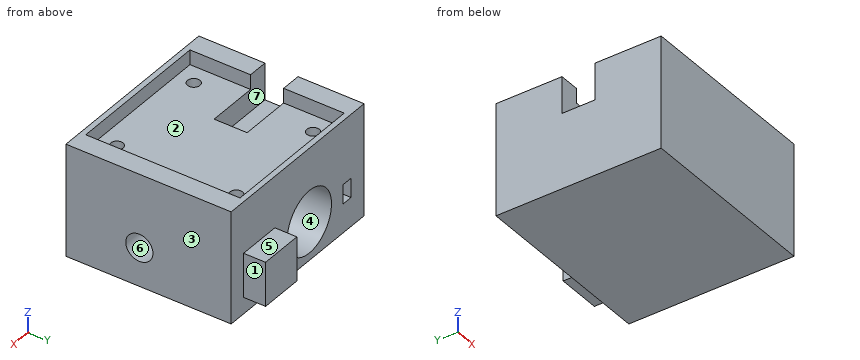
from build123d import *

# Parameters (mm, degrees)
BASE_R                        = 10.5
CUTLURE_TUBE_HOUSING_DEPTH    = 45
SKETCH1_W                     = 51
SKETCH1_H                     = 30.5
DETECTOR_LASER_HOUSING_DEPTH  = 45
CULTURE_SLOT_R                = 8.5
CULTURE_TUBE_SLOT_DEPTH       = 40
LASER_PORT_DEPTH              = 58.662812973
LASER_PORT_DEPTH_BACK         = 16
SKETCH3_R                     = 3.7
CUT_EXTRUDE3_REACH            = 59.663
CUT_EXTRUDE3_END_RADIUS       = 3.7
SKETCH4_W                     = 3
SKETCH4_H                     = 5.25
LED_DISPLAY_SCREW_HOLES_D     = 3.4
LED_DISPLAY_SCREW_HOLES_DEPTH = 20
SKETCH14_W                    = 40
SKETCH14_H                    = 42
CUT_EXTRUDE4_DEPTH            = 4
SKETCH16_W                    = 19.5
SKETCH16_H                    = 9
CUT_EXTRUDE6_DEPTH            = 10
SKETCH17_W                    = 12
SKETCH17_H                    = 12
BOSS_EXTRUDE3_DEPTH           = 6


with BuildPart() as part:
    # Base → Cutlure Tube Housing (new body)
    with BuildSketch(Plane(origin=(0, 0, 0), x_dir=(1, 0, 0), z_dir=(0, 1, 0))):
        with Locations(Location((0, 0, 0), (0, 0, 90))):
            Circle(BASE_R)
    extrude(amount=CUTLURE_TUBE_HOUSING_DEPTH)

    # Sketch1 → Detector+Laser Housing (add)
    with BuildSketch(Plane(origin=(0, 45, 0), x_dir=(1, 0, 0), z_dir=(0, 1, 0))):
        with Locations((4.5, -4.75)):
            Rectangle(SKETCH1_W, SKETCH1_H)
    extrude(amount=-DETECTOR_LASER_HOUSING_DEPTH)

    # Culture Slot → Culture Tube Slot (cut)
    with BuildSketch(Plane(origin=(0, 45, 0), x_dir=(1, 0, 0), z_dir=(0, 1, 0))):
        with Locations(Location((0, 0, 0), (0, 0, 270))):
            Circle(CULTURE_SLOT_R)
    extrude(amount=-CULTURE_TUBE_SLOT_DEPTH, mode=Mode.SUBTRACT)

    # Sketch3 → Laser Port (cut, two sides: drawn at the far end of the back side and taken through both)
    with BuildSketch(Plane(origin=(0, 0, 0), x_dir=(0, 0, -1), z_dir=(1, 0, 0)).offset(-LASER_PORT_DEPTH_BACK)):
        with Locations((0, 20)):
            Circle(SKETCH3_R)
    extrude(amount=LASER_PORT_DEPTH + LASER_PORT_DEPTH_BACK, mode=Mode.SUBTRACT)

    # Cut-Extrude3: up to this cylinder (the profile starts outside it)
    cut_extrude3_end = Plane(origin=(-14.5, 20, 0), z_dir=(1, 0, 0)) * Cylinder(CUT_EXTRUDE3_END_RADIUS, 127.726, mode=Mode.PRIVATE)
    # Sketch4 → Cut-Extrude3 (cut, up to the surface)
    with BuildSketch(Plane(origin=(0, 45, 0), x_dir=(1, 0, 0), z_dir=(0, 1, 0)), mode=Mode.PRIVATE) as cut_extrude3_sk1:
        with Locations((-14.5, 0)):
            Rectangle(SKETCH4_W, SKETCH4_H)
    cut_extrude3_tool1 = extrude(cut_extrude3_sk1.sketch, amount=-CUT_EXTRUDE3_REACH, mode=Mode.PRIVATE) - cut_extrude3_end
    add(cut_extrude3_tool1.solids().sort_by_distance((-14.5, 45, 0))[0], mode=Mode.SUBTRACT)

    # LED display Screw Holes
    with Locations(Plane.XY.offset(20)):
        with Locations((-10.25, 38.75), (-10.25, 6.25), (19.25, 38.75), (19.25, 6.25)):
            Hole(LED_DISPLAY_SCREW_HOLES_D / 2, depth=LED_DISPLAY_SCREW_HOLES_DEPTH)

    # Sketch14 → Cut-Extrude4 (cut)
    with BuildSketch(Plane.XY.offset(20)):
        with Locations((4.5, 22.5)):
            Rectangle(SKETCH14_W, SKETCH14_H)
    extrude(amount=-CUT_EXTRUDE4_DEPTH, mode=Mode.SUBTRACT)

    # Sketch16 → Cut-Extrude6 (cut)
    with BuildSketch(Plane.XY.offset(20)):
        with Locations((-11.25, 22.5)):
            Rectangle(SKETCH16_W, SKETCH16_H)
    extrude(amount=-CUT_EXTRUDE6_DEPTH, mode=Mode.SUBTRACT)

    # Sketch17 → Boss-Extrude3 (add)
    with BuildSketch(Plane(origin=(0, 45, 0), x_dir=(1, 0, 0), z_dir=(0, 1, 0))):
        with Locations((19.25, 0)):
            Rectangle(SKETCH17_W, SKETCH17_H)
    extrude(amount=BOSS_EXTRUDE3_DEPTH)


solid = part.part
Here's how the part is built. I have some questions about the finished solid (model axes, mm). Face numbers are marked on the shaded views. A direction names the side the tool comes from. Coordinates: 2 decimals unless noted, no trailing zeros. Order: outer loops, then holes, each group sorted by start corner. A loop starts at its lowest first (then second) coordinate and runs counter-clockwise, first axis right, second up. Notation, with made-up numbers: (60, 30) -> (72, 30) arc R27 cw to (72, 68) -> close; hole circle Ø1 at (36.25, 22.25). An arc over 180 degrees is marked (long way). Answer in a Markdown table with one row per item.
(1) I want a section at C-C on y = 6.25. List the corners of the cut face in (x, z) for me, then the cut area to 3 significant figures.
Answer key:
| item | result |
|---|---|
| outline | (-21, -10.5) -> (30, -10.5) -> (30, 20) -> (24.5, 20) -> (24.5, 16) -> (20.95, 16) -> (20.95, 0) -> (17.55, 0) -> (17.55, 16) -> (-8.55, 16) -> (-8.55, 0) -> (-11.95, 0) -> (-11.95, 16) -> (-15.5, 16) -> (-15.5, 20) -> (-21, 20) -> close; hole circle Ø17 at (0, 0) |
| area | 1,060 mm^2 |
(2) Thinking about a two-plate mould opening in Z: for the marked faces 4, 5, 6 and 7, which applies, +Z half, -Z half, draft (parallel to the pull), parting line (faces both ways), or undercut?
Answer key:
| item | result |
|---|---|
| face 4 | undercut |
| face 5 | +Z half |
| face 6 | undercut |
| face 7 | draft |
(3) On a 3-axis mill with a long thin cutter (end or side, diameter ignored), from which of +Z, -Z, +X, -X, +Y, -Y can I reach the whole of each face in a straight line? I mean the marked faces 1, 2 and 3. Say none if no direction works.
Answer key:
| item | result |
|---|---|
| face 1 | +Z, -Z, +X, +Y |
| face 2 | +Z |
| face 3 | +Z, -Z, +X, +Y, -Y |
(4) I want a section at D-D on y = 20. List the corners of the cut face in (x, z) for me, then the cut area to 3 significant figures.
Answer key:
| item | result |
|---|---|
| outline | (-21, -10.5) -> (30, -10.5) -> (30, -3.7) -> (7.65, -3.7) arc R8.5 cw to (-7.65, -3.7) -> (-16, -3.7) -> (-16, 3.7) -> (-7.65, 3.7) arc R8.5 cw to (7.65, 3.7) -> (30, 3.7) -> (30, 20) -> (24.5, 20) -> (24.5, 16) -> (-1.5, 16) -> (-1.5, 10) -> (-21, 10) -> close |
| area | 811 mm^2 |
(5) I want a section at B-B on x = 19.25. List the corners of the cut face in (y, z) for me.
Answer key:
| item | result |
|---|---|
| outline | (0, -10.5) -> (45, -10.5) -> (45, -6) -> (51, -6) -> (51, 6) -> (45, 6) -> (45, 20) -> (43.5, 20) -> (43.5, 16) -> (40.45, 16) -> (40.45, 0) -> (37.05, 0) -> (37.05, 16) -> (7.95, 16) -> (7.95, 0) -> (4.55, 0) -> (4.55, 16) -> (1.5, 16) -> (1.5, 20) -> (0, 20) -> close; hole circle Ø7.4 at (20, 0) |
(6) Please list where these lines run through material, in increasing order: probe 1 along X at (y, z) = (33, 0); probe 2 along Y at (x, z) = (19.25, 8.25); probe 3 along Z at (x, y) = (-14, 20).
Answer key:
| item | result |
|---|---|
| probe 1 | -21 to -16, -13 to -8.5, 8.5 to 30 |
| probe 2 | 0 to 4.55, 7.95 to 37.05, 40.45 to 45 |
| probe 3 | -10.5 to -3.7, 3.7 to 10 |
(7) Will these pins go through, and if not, where does the flat tip stop? pin 1 Ø8.5 at (x, z) = (-4, 3) entering from +Y; pin 2 Ø3 at (x, y) = (14, 41) entering from +Z; pin 3 Ø2 at (x, y) = (19.25, 38.75) entering from +Z.
Answer key:
| item | result |
|---|---|
| pin 1 | y = 45 |
| pin 2 | z = 16 |
| pin 3 | z = 0 |
(8) I want a section at A-A on z = 13. List the corners of the cut face in (x, y) for me.
Answer key:
| item | result |
|---|---|
| outline | (-21, 0) -> (30, 0) -> (30, 45) -> (-21, 45) -> (-21, 27) -> (-1.5, 27) -> (-1.5, 18) -> (-21, 18) -> close; hole circle Ø3.4 at (-10.25, 6.25); hole circle Ø3.4 at (-10.25, 38.75); hole circle Ø3.4 at (19.25, 6.25); hole circle Ø3.4 at (19.25, 38.75) |
